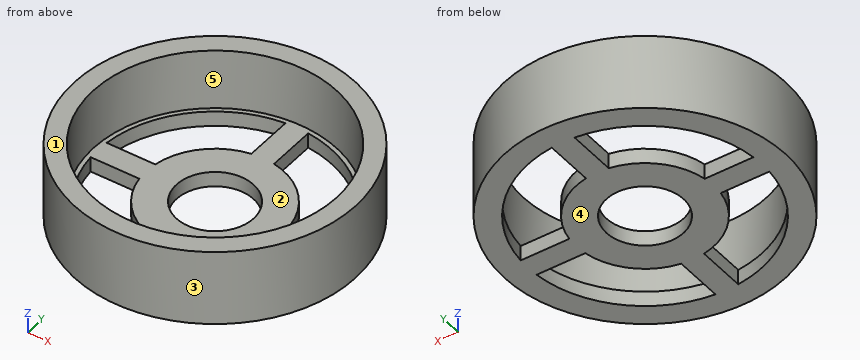
from build123d import *

# Parameters (mm, degrees)
ESBO_O1_R                = 16
ESBO_O1_R_2              = 5.075
RESSALTO_EXTRUS_O1_DEPTH = 2
ESBO_O2_R                = 18
ESBO_O2_R_2              = 16
RESSALTO_EXTRUS_O2_DEPTH = 10
CORTE_EXTRUS_O1_DEPTH    = 10
RESSALTO_EXTRUS_O3_START = -10
ESBO_O4_R                = 18.5
ESBO_O4_R_2              = 18
RESSALTO_EXTRUS_O3_DEPTH = 10


with BuildPart() as part:
    # Esboço1 → Ressalto-extrusão1 (new body)
    with BuildSketch(Plane.XY):
        Circle(ESBO_O1_R)
        Circle(ESBO_O1_R_2, mode=Mode.SUBTRACT)
    extrude(amount=RESSALTO_EXTRUS_O1_DEPTH)

    # Esboço2 → Ressalto-extrusão2 (add)
    with BuildSketch(Plane.XY):
        Circle(ESBO_O2_R)
        Circle(ESBO_O2_R_2, mode=Mode.SUBTRACT)
    extrude(amount=RESSALTO_EXTRUS_O2_DEPTH)

    # Esboço3 → Corte-extrusão1 (cut)
    with BuildSketch(Plane(origin=(0, 0, 0), x_dir=(-1, 0, 0), z_dir=(0, 0, -1))):
        with BuildLine():
            ThreePointArc((-1.5, -8.932222345), (-6.404474843, -6.404474843), (-8.932222345, -1.5))
            Line((-8.932222345, -1.5), (-15.344338178, -1.5))
            ThreePointArc((-15.344338178, -1.5), (-10.90180522, -10.90180522), (-1.5, -15.344338178))
            Line((-1.5, -15.344338178), (-1.5, -8.932222345))
        make_face()
        with BuildLine():
            ThreePointArc((8.932222345, -1.5), (6.404474843, -6.404474843), (1.5, -8.932222345))
            Line((1.5, -8.932222345), (1.5, -15.344338178))
            ThreePointArc((1.5, -15.344338178), (10.90180522, -10.90180522), (15.344338178, -1.5))
            Line((15.344338178, -1.5), (8.932222345, -1.5))
        make_face()
        with BuildLine():
            ThreePointArc((1.5, 8.932222345), (6.404474843, 6.404474843), (8.932222345, 1.5))
            Line((8.932222345, 1.5), (15.344338178, 1.5))
            ThreePointArc((15.344338178, 1.5), (10.90180522, 10.90180522), (1.5, 15.344338178))
            Line((1.5, 15.344338178), (1.5, 8.932222345))
        make_face()
        with BuildLine():
            ThreePointArc((-8.932222345, 1.5), (-6.404474843, 6.404474843), (-1.5, 8.932222345))
            Line((-1.5, 8.932222345), (-1.5, 15.344338178))
            ThreePointArc((-1.5, 15.344338178), (-10.90180522, 10.90180522), (-15.344338178, 1.5))
            Line((-15.344338178, 1.5), (-8.932222345, 1.5))
        make_face()
    extrude(amount=-CORTE_EXTRUS_O1_DEPTH, mode=Mode.SUBTRACT)

    # Esboço4 → Ressalto-extrusão3 (add)
    with BuildSketch(Plane.XY.offset(10).offset(RESSALTO_EXTRUS_O3_START)):
        Circle(ESBO_O4_R)
        Circle(ESBO_O4_R_2, mode=Mode.SUBTRACT)
    extrude(amount=RESSALTO_EXTRUS_O3_DEPTH)


solid = part.part
Model file for the job. Use its own axes, mm. Face numbers are marked on the shaded views. A direction names the side the tool comes from. Give positions to 0.01 mm unless a question says otherwise; leave off trailing zeros. Loops run counter-clockwise (first coordinate to the right, second up) from the corner with the lowest first, then second, coordinate; pieces in that order, holes last.
Item 1: Which spindle directions (+Z, -Z, +X, -X, +Y, -Y) get a long thin tool onto all of the face, cutting with end or side? Do the marked faces 4 and 5. Say none if no direction does.
Check values:
face 4: -Z, +X, -X, +Y, -Y
face 5: +Z
Item 2: Drop flat-ended pins along their axis: P1, Ø1.5, axis at x = -10, z = 5.5, coming from the +Y side; P2, Ø13, axis at x = 0, y = 0, coming from the -Z side; P3, Ø6, axis at y = -10, z = 8, coming from the -X side; P4, Ø1, axis at y = -12, z = 1, coming from the +X side. Give the stop position or say it passes through.
Check values:
P1: stops at y = 16.02
P2: stops at z = 0
P3: stops at x = -17.12
P4: stops at x = 14.49
Item 3: Slice it at A-A (y = 0). Write the cut outline in (x, z) (3 decimals), plus the area to 3 significant figures.
Check values:
outline: (-18.5, 0) - (-5.075, 0) - (-5.075, 2) - (-16, 2) - (-16, 10) - (-18.5, 10) - close; (5.075, 0) - (18.5, 0) - (18.5, 10) - (16, 10) - (16, 2) - (5.075, 2) - close
area: 93.7 mm2
Item 4: Slice it at D-D (y = -8.5). Write the cut outline in (x, z), plus the area to 3 significant figures.
Check values:
outline: (-16.43, 0) - (-12.86, 0) - (-12.86, 2) - (-13.56, 2) - (-13.56, 10) - (-16.43, 10) - close; (-3.13, 0) - (3.13, 0) - (3.13, 2) - (-3.13, 2) - close; (12.86, 0) - (16.43, 0) - (16.43, 10) - (13.56, 10) - (13.56, 2) - (12.86, 2) - close
area: 72.8 mm2
Item 5: Drill centre lines: line 1 along Y through (x, z) = (0, 5); line 2 along Z through (x, y) = (8, -2); line 3 along Y through (x, z) = (0, 0.8) (3 decimals). Where is each one in solid material? Low to high.
Check values:
line 1: y = -18.5 to -16, 16 to 18.5
line 2: z = 0 to 2
line 3: y = -18.5 to -5.075, 5.075 to 18.5
Item 6: Slice it at B-B (z = 0.75). Write the cut outline in (x, y) (3 decimals).
Check values:
outline: circle Ø37 at (0, 0); hole (-15.344, -1.5) arc R15.417 ccw to (-1.5, -15.344) - (-1.5, -8.932) arc R9.057 cw to (-8.932, -1.5) - close; hole (-15.344, 1.5) - (-8.932, 1.5) arc R9.057 cw to (-1.5, 8.932) - (-1.5, 15.344) arc R15.417 ccw to start; hole circle Ø10.15 at (0, 0); hole (1.5, -15.344) arc R15.417 ccw to (15.344, -1.5) - (8.932, -1.5) arc R9.057 cw to (1.5, -8.932) - close; hole (1.5, 8.932) arc R9.057 cw to (8.932, 1.5) - (15.344, 1.5) arc R15.417 ccw to (1.5, 15.344) - close
Item 7: Mould opens along Y. For the marked faces 1, 2 and 3 say: +Y half, -Y half, draft (parallel to the pull), parting line (faces both ways), or undercut.
Check values:
face 1: draft
face 2: undercut
face 3: parting line
